Work out the finished part from the listing and answer in its coordinate system (mm). A direction names the side the tool comes from. Round coordinates to 2 decimals unless told otherwise and drop trailing zeros. Write each loop counter-clockwise with the first axis right and the second up, starting at its lowest first coordinate (ties: lowest second). Pieces come first, ordered by that corner, then holes. Notation, with made-up numbers: (73.25, 40) -> (95.25, 40) arc R13 cw to (95.25, 49) -> close; hole circle Ø8 at (72.25, 31.25). An arc over 180 degrees is marked (long way). One line per question, with ' | ' between items. Start each with the question number.
```python
from build123d import *

# Parameters (mm, degrees)
BOSS_EXTRUDE1_DEPTH     = 27.7
SKETCH2_R               = 1.6
CUT_EXTRUDE1_DEPTH      = 6.4
MIRROR1_START           = 25
MIRROR1_OUTLINE_R       = 1.6
MIRROR1_DEPTH           = 4
BOSS_EXTRUDE2_DEPTH     = 27.7
CUT_EXTRUDE2_DEPTH      = 8
CUT_EXTRUDE2_DEPTH_BACK = 8
SKETCH4_R               = 1.6
CUT_EXTRUDE3_DEPTH      = 8


# Read off the part's stored shape, not the designer's step: Mirror1
with BuildPart() as part:
    # Sketch1 → Boss-Extrude1 (new body)
    with BuildSketch(Plane.XY):
        Polygon((-34, 29), (34, 29), (34, -29), (30, -25), (30, 25), (-30, 25), align=None)
    extrude(amount=BOSS_EXTRUDE1_DEPTH)

    # Sketch2 → Cut-Extrude1 (cut)
    with BuildSketch(Plane(origin=(34, 0, 0), x_dir=(0, 0, -1), z_dir=(1, 0, 0))):
        with Locations((-3.5, -15.2)):
            Circle(SKETCH2_R)
        with Locations((-3.5, 15.2)):
            Circle(SKETCH2_R)
    extrude(amount=-CUT_EXTRUDE1_DEPTH, mode=Mode.SUBTRACT)

    # Mirror1 outline → Mirror1 (cut)
    with BuildSketch(Plane(origin=(0, 0, 0), x_dir=(1, 0, 0), z_dir=(0, 1, 0)).offset(MIRROR1_START)):
        with Locations((20.2, -3.5)):
            Circle(MIRROR1_OUTLINE_R)
    mirror1 = extrude(amount=MIRROR1_DEPTH, mode=Mode.SUBTRACT)

    # Mirror2: Mirror1 across plane
    add(mirror1.mirror(Plane(origin=(0, 0, 0), x_dir=(0, 0, 1), z_dir=(1, 0, 0))), mode=Mode.SUBTRACT)

    # Sketch3 → Boss-Extrude2 (add)
    with BuildSketch(Plane.XY.offset(27.7)):
        Polygon((-34, 29), (-41.778174593, 36.778174593), (-35.778174593, 36.778174593), (-28, 29), align=None)
        Polygon((34, -29), (41.778174593, -36.778174593), (41.778174593, -30.778174593), (34, -23), align=None)
    extrude(amount=-BOSS_EXTRUDE2_DEPTH)

    # Sketch4 → Cut-Extrude2 (cut, two sides: drawn at the far end of the back side and taken through both)
    with BuildSketch(Plane(origin=(0.5, 0.5, 0), x_dir=(0, 0, -1), z_dir=(0.7071067811865475, 0.7071067811865477, 0)).offset(-CUT_EXTRUDE2_DEPTH_BACK)):
        with Locations(Location((-4, 45.805086528, 0), (0, 0, 90))):
            Circle(SKETCH4_R)
        with Locations(Location((-23.7, 45.805086528, 0), (0, 0, 90))):
            Circle(SKETCH4_R)
        with Locations(Location((-23.7, -45.794913472, 0), (0, 0, 90))):
            Circle(SKETCH4_R)
        with Locations(Location((-4, -45.794913472, 0), (0, 0, 90))):
            Circle(SKETCH4_R)
    extrude(amount=CUT_EXTRUDE2_DEPTH + CUT_EXTRUDE2_DEPTH_BACK, mode=Mode.SUBTRACT)

    # Sketch5 → Cut-Extrude3 (cut)
    with BuildSketch(Plane.XZ.offset(-25)):
        with BuildLine():
            Line((-1.8, 13.9), (1.8, 13.9))
            ThreePointArc((1.8, 13.9), (2.4, 13.3), (1.8, 12.7))
            Line((1.8, 12.7), (-1.8, 12.7))
            ThreePointArc((-1.8, 12.7), (-2.4, 13.3), (-1.8, 13.9))
        make_face()
    extrude(amount=-CUT_EXTRUDE3_DEPTH, mode=Mode.SUBTRACT)


solid = part.part
```
(1) Given pin 1 Ø1 at (x, z) = (-10.5, 10.5) entering from -Y; pin 2 Ø5 at (y, z) = (-11, 23) entering from +X; pin 3 Ø8.5 at (x, z) = (-7, 17) entering from +Y; pin 4 Ø3 at (x, y) = (0.5, 26.5) entering from -Z, each flat-ended and moving along its own axis, determine where each tip first touches the part or whether it passes through.
(2) A cutting plane is placed at C-C, the plane z = 11. Determine the outline of the cut face in (x, y), then the cut area to 3 significant figures.
(3) A cutting plane is placed at D-D, the plane y = -6. Determine the outline of the cut face in (x, z), then the cut area to 3 significant figures.
(4) For faces 5 (the flat face through (34, 3, 14)), 6 (the flat face through (30, 0, 14)), 7 (the cylindrical face through (32.03, 13.78, 2.76)), 8 (the flat face through (0, 27, 13.9)), 9 (the cylindrical face through (-32.51, 30.47, 22.73)), determine the directions among +Z, -Z, +X, -X, +Y, -Y from which every point of the face is accessible in a straight line to the end or side of a thin tool.
(5) Consider L1, parallel to Z at x = 32, y = -15; L2, parallel to X at y = 26.8, z = 3.5; L3, parallel to Y at x = 32.15, z = 3.5. Determine where each line is inside the solid, lowest interval first.
(6) A cutting plane is placed at B-B, the plane x = -20.2. Determine the outline of the cut face in (y, z), then the cut area to 3 significant figures.
(7) The mould has two halves that part along Z. Classify faces 1 (the flat face through (13, 27, 27.7)), 2 (the flat face through (36, -31, 14)), 3 (the cylindrical face through (32.03, -16.76, 3.85)), 4 (the cylindrical face through (36.61, -28.65, 22.14)): +Z half, -Z half, draft (parallel to the pull), parting line (faces both ways), or undercut.
(8) A cutting plane is placed at A-A, the plane y = -15.2. Determine the outline of the cut face in (x, z).
Returned:
1) pin 1: y = 25 | pin 2: x = 34 | pin 3: y = 29 | pin 4: z = 0
2) outline: (-41.78, 36.78) -> (-30, 25) -> (30, 25) -> (30, -25) -> (41.78, -36.78) -> (41.78, -30.78) -> (34, -23) -> (34, 29) -> (-28, 29) -> (-35.78, 36.78) -> close | area: 565 mm2
3) outline: (30, 0) -> (34, 0) -> (34, 27.7) -> (30, 27.7) -> close | area: 111 mm2
4) face 5: +Z, -Z, +X, +Y | face 6: +Z, -Z, -X, -Y | face 7: +X, -X | face 8: +Y, -Y | face 9: none
5) L1: 0 to 1.91, 5.09 to 27.7 | L2: -31.8 to -21.8, -18.6 to 18.6, 21.8 to 34 | L3: -27.15 to -16.8, -13.6 to 13.6, 16.8 to 29
6) outline: (25, 0) -> (29, 0) -> (29, 1.9) -> (25, 1.9) -> close; (25, 5.1) -> (29, 5.1) -> (29, 27.7) -> (25, 27.7) -> close | area: 98.0 mm2
7) face 1: +Z half | face 2: draft | face 3: undercut | face 4: undercut
8) outline: (30, 0) -> (34, 0) -> (34, 1.9) -> (30, 1.9) -> close; (30, 5.1) -> (34, 5.1) -> (34, 27.7) -> (30, 27.7) -> close
